Autodesk Inventor part; units mm, degrees
ref_plane "YZ Plane" through (0, 0, 0) normal (1, 0, 0) x (0, 1, 0)
ref_plane "XZ Plane" through (0, 0, 0) normal (0, 1, 0) x (-1, 0, 0)
ref_plane "XY Plane" through (0, 0, 0) normal (0, 0, 1) x (1, 0, 0)
sketch "Sketch1" plane through (0, 0, 0) normal (0, 1, 0) x (-1, 0, 0)
  circle A0 centre (0, 0) radius 13
  circle A1 centre (0, 0) radius 15.5
  circle A2 centre (0, 18.5) radius 2.75
  circle A3 centre (0, -18.5) radius 2.75
  line L0 (0, 18.5) -> (0, -18.5)
  line L1 (7.5, 22.5) -> (-7.5, 22.5)
  line L2 (-7.5, 22.5) -> (-7.5, 13)
  line L3 (-7.5, 13) -> (7.5, 13)
  line L4 (7.5, 13) -> (7.5, 22.5)
  line L5 (0, 22.5) -> (7.5, 18.5)
  line L6 (7.5, 18.5) -> (7.5, 13.5647)
  line L7 (0, 22.5) -> (-7.5, 18.5)
  line L8 (-7.5, 18.5) -> (-7.5, 13.5647)
  line L9 (13, 0) -> (-13, 0) construction
  circle A4 centre (0, -18.5) radius 2.75
  line L10 (7.5, -22.5) -> (-7.5, -22.5)
  line L11 (-7.5, -22.5) -> (-7.5, -13)
  line L12 (7.5, -13) -> (7.5, -22.5)
  line L13 (0, -22.5) -> (7.5, -18.5)
  line L14 (0, -22.5) -> (-7.5, -18.5)
  point P0 (-7.5, -13.5647)
  point P1 (7.5, -13.5647)
  dimension "d0" = 26
  dimension "d1" = 2.5
  dimension "d2" = 5.5
  dimension "d3" = 5.5
  dimension "d4" = 37
  dimension "d5" = 15
  dimension "d6" = 4
extrude "Extrusion1" add sketch "Sketch1" along normal blind 5 contours A0 L3 L4 A1 L0 | L3 L2 A1 L0 | A0 L0 A1 L2 L3 | L0 A1 L4 L3 | A1 L2 L7 L5 L4 | A1 L12 L13 L14 L11
sketch "Sketch2" plane through (0, 0, 0) normal (0, -1, 0) x (1, 0, 0)
  line L0 (7.5, -18.5) -> (0, -22.5)
  line L1 (0, -22.5) -> (-15.5, -22.5)
  line L2 (-15.5, -22.5) -> (-15.5, 22.5)
  line L3 (-15.5, 22.5) -> (0, 22.5)
  arc A0 (-7.5, 13.5647) -> (-7.5, -13.5647) centre (0, 0) ccw
  line L4 (-7.5, 13.5647) -> (-7.5, 18.5)
  line L5 (0, 22.5) -> (-7.5, 18.5)
  line L6 (-7.5, 18.5) -> (-7.5, 13.5647)
  arc A1 (-7.5, 13.5647) -> (-15.5, 0) centre (0, 0) ccw
  line L7 (0, -22.5) -> (-7.5, -18.5)
  line L8 (0, -22.5) -> (-7.5, -18.5)
  line L9 (-7.5, -18.5) -> (-7.5, -13.5647)
  line L10 (-7.5, -18.5) -> (-7.5, -13.5647)
  arc A2 (-7.5, 13.5647) -> (-7.5, -13.5647) centre (0, 0) ccw
  point P0 (-15.5, 0)
extrude "Extrusion2" add sketch "Sketch2" against normal up to surface (5 mm away)
sketch "Sketch4" plane through (0, 5, 0) normal (0, 1, 0) x (1, 0, 0)
  arc A0 (7.5, -13.5647) -> (7.5, 13.5647) centre (0, 0) ccw
  arc A1 (7.5, -13.5647) -> (7.5, 13.5647) centre (0, 0) ccw
  line L0 (7.5, 13.5647) -> (7.5, 18.5)
  line L1 (7.5, 13.5647) -> (-5.5, 13.5647)
  line L2 (-5.5, 13.5647) -> (-5.5, 22.5742)
  line L3 (-5.5, 22.5742) -> (-15.5, 22.5742)
  line L4 (-15.5, -22.5) -> (-15.5, 22.5)
  line L5 (-15.5, 22.5742) -> (-15.5, -22.5)
  line L6 (0, -22.5) -> (-15.5, -22.5)
  line L7 (-15.5, -22.5) -> (-5.5, -22.5)
  line L8 (-5.5, -22.5) -> (-5.5, -13.5647)
  line L9 (-5.5, -13.5647) -> (7.5, -13.5647)
  line L10 (7.5, -18.5) -> (7.5, -13.5647)
  circle A2 centre (0, 0) radius 9.5
  point P0 (-15.5, -30.5)
  point P1 (-15.5, 30.5)
  point P2 (-10, -22.5)
  point P3 (-15.5, -22.5)
  point P4 (-5.5, -22.5)
  point P5 (-5.5, -22.5)
  dimension "d21" = 13
  dimension "d22" = 13
  dimension "d23" = 19
extrude "Extrusion4" add sketch "Sketch4" along normal blind 5.5
sketch "Sketch5" plane through (-15.5, 0, -22.5) normal (-1, 0, 0) x (0, 0, 1)
  line L0 (45, 0) -> (45, 5)
  line L1 (45, 0) -> (53, 0)
  line L2 (53, 0) -> (53, 10.5)
  line L3 (53, 10.5) -> (45, 10.5)
  line L4 (45, 10.5) -> (45, 0)
  line L5 (4, 0) -> (0, 0)
  line L6 (0, 0) -> (-8, 0)
  line L7 (-8, 0) -> (-8, 10.5)
  line L8 (-8, 10.5) -> (0, 10.5)
  line L9 (0, 10.5) -> (0, 0)
  line L10 (-0.0742, 10.5) -> (45, 10.5)
  line L11 (-4, 3.25) -> (-4, 7.25) construction
  line L12 (-1.5, 3.25) -> (-1.5, 7.25)
  line L13 (-6.5, 7.25) -> (-6.5, 3.25)
  arc A0 (-6.5, 3.25) -> (-1.5, 3.25) centre (-4, 3.25) ccw
  arc A1 (-1.5, 7.25) -> (-6.5, 7.25) centre (-4, 7.25) ccw
  line L14 (49, 3.25) -> (49, 7.25) construction
  line L15 (51.5, 3.25) -> (51.5, 7.25)
  line L16 (46.5, 7.25) -> (46.5, 3.25)
  arc A2 (46.5, 3.25) -> (51.5, 3.25) centre (49, 3.25) ccw
  arc A3 (51.5, 7.25) -> (46.5, 7.25) centre (49, 7.25) ccw
  point P0 (22.5, 0)
  point P1 (49, 10.5)
  point P2 (0, 5.25)
  point P3 (-4, 5.25)
  point P4 (-4, 0)
  point P5 (-6.5, 5.25)
  point P6 (49, 5.25)
  point P7 (46.5, 5.25)
  point P8 (45, 5.25)
  dimension "d26" = 8
  dimension "d27" = 8
  dimension "d28" = 0
  dimension "d29" = 4
  dimension "d30" = 5
  dimension "d31" = 4
  dimension "d32" = 5
extrude "Extrusion5" add sketch "Sketch5" against normal blind 8
properties part number "clock_part1"
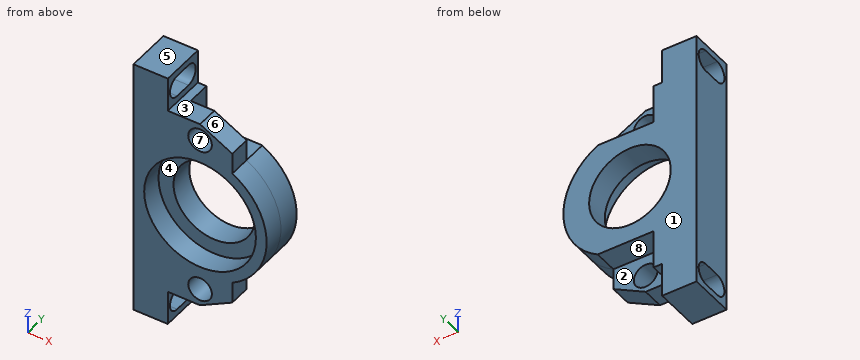
Geometry: final body of the model. Coordinates: model frame, mm. Face numbers are marked on the shaded views. A direction names the side the tool comes from. Round coordinates to 2 decimals unless told otherwise and drop trailing zeros. Loops run counter-clockwise (first coordinate to the right, second up) from the corner with the lowest first, then second, coordinate; pieces in that order, holes last.
Q1. Section C-C on x = -2. Return loops of the section in (y, z), plus the area to 3 significant figures.
Q2. Material intervals for L1, parallel to Z at x = 0, y = 1.4; L2, parallel to X at y = 6.8, z = 0; L3, parallel to Z at x = -10.5, y = 1.5, sorted ascending.
Q3. Section B-B on z = -26.5. Return loops of the section in (x, y), plus the area to 3 significant figures.
Q4. Section A-A on y = 6.5. Return loops of the section in (x, z).
Q5. Access query for the marked faces 1, 2, 3, 4 and 5. Directions: +Z, -Z, +X, -X, +Y, -Y. A direction counts if a zero-diameter tool reaches every point of the face in a straight line with its end or side. Return the directions, or none.
Q6. Section D-D on y = 1.5. Return loops of the section in (x, z).
Q7. Pull-direction query (X, two-part tool) for the marked faces 6, 7 and 8; classes: released by +X, released by -X, zero draft, split by the parting line, or undercut.
Q8. Pin query (flat end, axial travel): P1, Ø10, axis at x = 12, z = 1, coming from the -Y side; P2, Ø6, axis at x = 12, y = 5, coming from the -Z side; P3, Ø6, axis at x = 4, y = 7, coming from the -Z side; P4, Ø2.5, axis at x = 2, z = 16.5, coming from the +Y side. Return the tip coordinate at first contact, or that it passes through.
Evaluation:
1. outline: (0, -22.5) - (5, -22.5) - (5, -20.39) - (0, -20.39) - close; (0, -16.61) - (5, -16.61) - (5, -13.56) - (10.5, -13.56) - (10.5, -9.29) - (5, -9.29) - (5, -12.85) - (0, -12.85) - close; (0, 12.85) - (5, 12.85) - (5, 9.29) - (10.5, 9.29) - (10.5, 13.56) - (5, 13.56) - (5, 16.61) - (0, 16.61) - close; (0, 20.39) - (5, 20.39) - (5, 22.5) - (0, 22.5) - close
1. area: 106 mm2
2. L1: z = -22.5 to -21.25, -15.75 to -13, 13 to 15.75, 21.25 to 22.5
2. L2: x = -15.5 to -9.5, 9.5 to 15.5
2. L3: z = -30.5 to -28.29, -24.71 to -7.66, 7.66 to 24.71, 28.29 to 30.5
3. outline: (-15.5, 0) - (-7.5, 0) - (-7.5, 0.75) - (-15.5, 0.75) - close; (-15.5, 9.75) - (-7.5, 9.75) - (-7.5, 10.5) - (-15.5, 10.5) - close
3. area: 12.0 mm2
4. outline: (-15.5, -30.5) - (-7.5, -30.5) - (-7.5, -29) - (-15.5, -29) - close; (-15.5, -24) - (-7.5, -24) - (-7.5, -22.57) - (-5.5, -22.57) - (-5.5, -13.56) - (7.5, -13.56) arc R15.5 ccw to (7.5, 13.56) - (-5.5, 13.56) - (-5.5, 22.5) - (-7.5, 22.5) - (-7.5, 24) - (-15.5, 24) - close; (-15.5, 29) - (-7.5, 29) - (-7.5, 30.5) - (-15.5, 30.5) - close; hole circle Ø19 at (0, 0)
5. face 1: +Z, -Z, +X, -X, +Y
5. face 2: -Z, +X, +Y
5. face 3: +Z, +X, +Y, -Y
5. face 4: -Y
5. face 5: +Z, +X, -X, +Y, -Y
6. outline: (-15.5, -30.5) - (-7.5, -30.5) - (-7.5, -28.29) - (-15.5, -28.29) - close; (-15.5, -24.71) - (-7.5, -24.71) - (-7.5, -22.5) - (0, -22.5) - (7.5, -18.5) - (7.5, -13.56) arc R15.5 ccw to (7.5, 13.56) - (7.5, 18.5) - (0, 22.5) - (-7.5, 22.5) - (-7.5, 24.71) - (-15.5, 24.71) - close; (-15.5, 28.29) - (-7.5, 28.29) - (-7.5, 30.5) - (-15.5, 30.5) - close; hole circle Ø26 at (0, 0); hole circle Ø5.5 at (0, -18.5); hole circle Ø5.5 at (0, 18.5)
7. face 6: released by +X
7. face 7: undercut
7. face 8: zero draft
8. P1: stops at y = 0
8. P2: stops at z = -12.62
8. P3: stops at z = -21.56
8. P4: stops at y = 5
